Answer from the drawing. Dimensions are ordinates in mm from the lowest x, y and z of the part. A direction names the side the tool comes from. Coordinates: 2 decimals unless noted, no trailing zeros. Write each loop counter-clockwise with the first axis right and the second up, starting at its lowest first coordinate (ties: lowest second). Pieces come first, ordered by that corner, then holes. Notation, with made-up numbers: (43, 37.5) - (102, 37.5) arc R17 ccw to (102, 58.5) - close; hole circle Ø5 at (-23.75, -0.75). An arc over 180 degrees is marked (long way). Return JSON: item names as keys, results as strings.
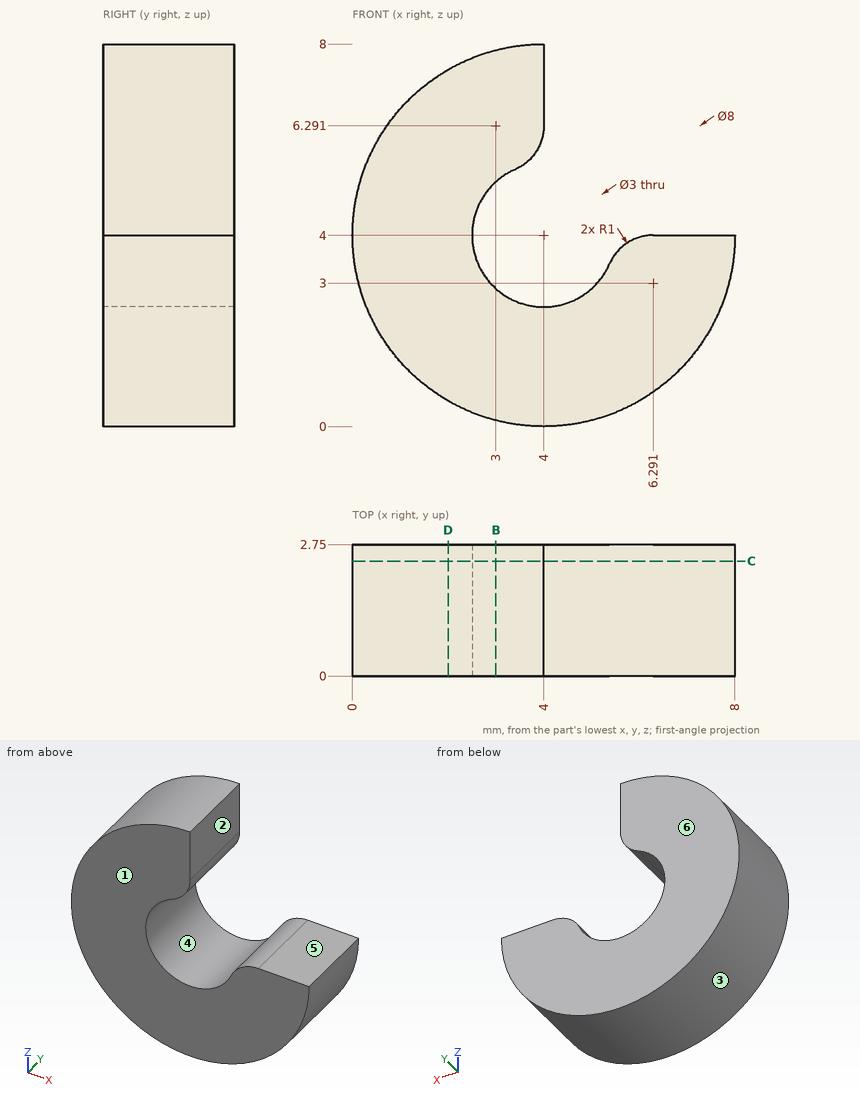
(1) Which of the six approach directions +Z, -Z, +X, -X, +Y, -Y give full straight-line access (tool end or side, diameter ignored) to the marked faces 1 and 2?
Answer:
{"face 1": "+Z, -Z, +X, -X, -Y", "face 2": "+Z, +X, +Y, -Y"}
(2) A cutting plane is placed at C-C (y = 2.4). Determine the outline of the cut face in (x, z) (1 decimal), and give its area (3 significant figures).
Answer:
{"outline": "(3.4, 5.4) arc R1 ccw to (4, 6.3) - (4, 8) arc R4 ccw (long way) to (8, 4) - (6.3, 4) arc R1 ccw to (5.4, 3.4) arc R1.5 cw (long way) to start", "area": "32.2 mm²"}
(3) A cutting plane is placed at B-B (x = 3). Determine the outline of the cut face in (y, z).
Answer:
{"outline": "(0, 0.13) - (2.75, 0.13) - (2.75, 2.88) - (0, 2.88) - close; (0, 5.12) - (2.75, 5.12) - (2.75, 7.87) - (0, 7.87) - close"}
(4) A cutting plane is placed at D-D (x = 2). Determine the outline of the cut face in (y, z).
Answer:
{"outline": "(0, 0.54) - (2.75, 0.54) - (2.75, 7.46) - (0, 7.46) - close"}
(5) Straight lines are drawn through the part: line 1 (X direction, y = 2.25, z = 3.25); line 2 (Z direction, x = 3.5, y = 0.55) (1 decimal). For each, find the intervals that lie inside material, in ascending order. Write a range as from..to.
Answer:
{"line 1": "0.07..2.7, 5.3..7.93", "line 2": "0..2.6, 5.4..8"}
(6) A flat-ended cylindrical pin translates along its axis: P1, Ø0.5, axis at x = 7.5, y = 1, coming from the +Z side. Find the tip coordinate at first contact, or state that the pin passes through.
Answer:
{"P1": "z = 4"}
(7) Determine the mould class of the marked faces 3, 4, 5 and 6 for opening direction Z: +Z half, -Z half, draft (parallel to the pull), parting line (faces both ways), or undercut.
Answer:
{"face 3": "parting line", "face 4": "undercut", "face 5": "+Z half", "face 6": "draft"}
